Part model, mm, in its own coordinate system. A direction names the side the tool comes from. Give positions to 0.01 mm unless a question says otherwise; leave off trailing zeros. Order: outer loops, then holes, each group sorted by start corner. A loop starts at its lowest first (then second) coordinate and runs counter-clockwise, first axis right, second up.
1. Probe line 1 (Y direction, x = 53, z = 2); line 2 (X direction, y = -2.5, z = -10); line 3 (Y direction, x = 30.5, z = 10.75). List the from-to ranges inside material, lowest first.
2. Mould opens along X. For faces 3 (the flat face through (380, 3, 0)), 4 (the flat face through (374, -3.95, 0)), 5 (the flat face through (0, 3, 0)), 6 (the cylindrical face through (370, -3, 0)) say: +X half, -X half, draft (parallel to the pull), parting line (faces both ways), or undercut.
3. Which spindle directions (+Z, -Z, +X, -X, +Y, -Y) get a long thin tool onto all of the face, cutting with end or side? Do faces 1 (the cylindrical face through (170, -3, 0)), 2 (the cylindrical face through (145.12, 1.43, -13.68)). Say none if no direction does.
4. Slice it at B-B on y = -1.25. List the corners of the cut face in (x, z), and give its area (3 significant figures).
5. Drop flat-ended pins along their axis: pin 1 Ø2 at (x, z) = (232.5, -0.5) entering from -Y; pin 2 Ø7.5 at (x, z) = (317, -10) entering from -Y; pin 3 Ø1.5 at (x, y) = (316.5, 2.5) entering from -Z. Give the stop position or say it passes through.
6. Slice it at A-A on x = 122.5. List the corners of the cut face in (y, z), and give its area (3 significant figures).
from build123d import *

# Parameters (mm, degrees)
EXTRUDE_1_DEPTH     = 380
CUT_EXTRUDE_1_DEPTH = 390
CUT_EXTRUDE_2_DEPTH = 5.9


with BuildPart() as part:
    # 草图2 → 凸台-拉伸1 (new body)
    with BuildSketch(Plane(origin=(0, 0, 0), x_dir=(0, 0, -1), z_dir=(1, 0, 0))):
        with BuildLine():
            Line((-10, 3.95), (10, 3.95))
            ThreePointArc((10, 3.95), (13.95, 0), (10, -3.95))
            Line((10, -3.95), (-10, -3.95))
            ThreePointArc((-10, -3.95), (-13.95, 0), (-10, 3.95))
        make_face()
    extrude(amount=EXTRUDE_1_DEPTH)

    # 草图3 → 切除-拉伸1 (cut)
    with BuildSketch(Plane.ZY):
        with BuildLine():
            Line((2.5, -2.5), (-2.5, -2.5))
            ThreePointArc((-2.5, -2.5), (-5, 0), (-2.5, 2.5))
            Line((-2.5, 2.5), (2.5, 2.5))
            ThreePointArc((2.5, 2.5), (5, 0), (2.5, -2.5))
        make_face()
    extrude(amount=-CUT_EXTRUDE_1_DEPTH, mode=Mode.SUBTRACT)

    # 草图5 → 切除-拉伸2 (cut)
    with BuildSketch(Plane.XZ.offset(3.95)):
        with BuildLine():
            Line((197.278769414, 27.278769414), (342.721230586, 27.278769414))
            ThreePointArc((342.721230586, 27.278769414), (370, 0), (342.721230586, -27.278769414))
            Line((342.721230586, -27.278769414), (197.278769414, -27.278769414))
            ThreePointArc((197.278769414, -27.278769414), (170, 0), (197.278769414, 27.278769414))
        make_face()
    extrude(amount=-CUT_EXTRUDE_2_DEPTH, mode=Mode.SUBTRACT)


solid = part.part
Data:
1. line 1: y = -3.95 to -2.5, 2.5 to 3.95
1. line 2: x = 0 to 171.9, 368.1 to 380
1. line 3: y = -3.88 to 3.88
2. face 3: +X half
2. face 4: draft
2. face 5: -X half
2. face 6: undercut
3. face 1: -Y
3. face 2: -Z, +X, -X
4. outline: (0, -13.75) - (173.72, -13.75) arc R27.28 cw to (170.4, -4.67) - (0, -4.67) - close; (0, 4.67) - (170.4, 4.67) arc R27.28 cw to (173.72, 13.75) - (0, 13.75) - close; (366.28, -13.75) - (380, -13.75) - (380, -4.67) - (369.6, -4.67) arc R27.28 cw to start; (366.28, 13.75) arc R27.28 cw to (369.6, 4.67) - (380, 4.67) - (380, 13.75) - close
4. area: 3,330 mm2
5. pin 1: stops at y = 2.5
5. pin 2: stops at y = 1.95
5. pin 3: stops at z = -13.44
6. outline: (-3.95, -10) arc R3.95 ccw to (3.95, -10) - (3.95, 10) arc R3.95 ccw to (-3.95, 10) - close; hole (-2.5, -2.5) arc R2.5 ccw to (2.5, -2.5) - (2.5, 2.5) arc R2.5 ccw to (-2.5, 2.5) - close
6. area: 162 mm2
